The listing builds one solid part. Answer for the finished solid, in the listing's coordinates (mm). Face numbers are marked on the shaded views. A direction names the side the tool comes from. Round coordinates to 2 decimals unless told otherwise and drop trailing zeros. Write each loop counter-clockwise with the first axis right and the second up, starting at its lowest first coordinate (ties: lowest second). Pieces come first, ordered by that corner, then holes.
(1) For the marked faces 1 and 2, determine the directions among +Z, -Z, +X, -X, +Y, -Y from which every point of the face is accessible in a straight line to the end or side of a thin tool.
(2) Each of these flat-tipped pins is pushed along its axis until it touches: pin 1 Ø3 at (x, z) = (-27, -23.5) entering from -Y; pin 2 Ø1.5 at (x, y) = (-22.5, -10) entering from -Z; pin 3 Ø4 at (x, y) = (4.5, -9) entering from -Z; pin 4 Ø8 at (x, z) = (1.5, 0.5) entering from +Y. Where does it stop, or does it pass through?
(3) A cutting plane is placed at B-B, the plane x = 0. Give the vertices of the cut face in (y, z).
(4) A cutting plane is placed at D-D, the plane y = -12. Give the vertices of the cut face in (x, z).
(5) A cutting plane is placed at A-A, the plane z = 0. Give the vertices of the cut face in (x, y), and give its area (3 significant figures).
(6) Find the intervals of material crossed by probe 1 along X at (y, z) = (-2.5, 8); probe 2 along Y at (x, z) = (-21, 17); probe 3 along X at (y, z) = (1.25, -0.5), in increasing order.
(7) A cutting plane is placed at C-C, the plane y = -3. Give the vertices of the cut face in (x, z), and give its area (3 significant figures).
(8) The mould has two halves that part along X. Classify the marked faces 3, 4 and 5: +X half, -X half, draft (parallel to the pull), parting line (faces both ways), or undercut.
from build123d import *

# Parameters (mm, degrees)
CROQUIS1_R              = 35
SALIENTE_EXTRUIR1_DEPTH = 5
CROQUIS2_R              = 24.5
SALIENTE_EXTRUIR2_DEPTH = 15
CROQUIS3_R              = 6.85
SALIENTE_EXTRUIR3_DEPTH = 30
CROQUIS4_R              = 2
CORTAR_EXTRUIR1_DEPTH   = 10
MATRIZC1_COUNT          = 6
CORTAR_EXTRUIR2_START   = -30
CORTAR_EXTRUIR2_DEPTH   = 30
CUT_EXTRUDE1_START      = -40
CUT_EXTRUDE1_DEPTH      = 40
SKETCH2_R               = 5
CUT_EXTRUDE2_DEPTH      = 7
SKETCH3_R               = 3
CUT_EXTRUDE3_DEPTH      = 52.176166328


with BuildPart() as part:
    # Croquis1 → Saliente-Extruir1 (new body)
    with BuildSketch(Plane(origin=(0, 0, 0), x_dir=(1, 0, 0), z_dir=(0, 1, 0))):
        with Locations(Location((0, 0, 0), (0, 0, 270))):
            Circle(CROQUIS1_R)
    extrude(amount=SALIENTE_EXTRUIR1_DEPTH)

    # Croquis2 → Saliente-Extruir2 (add)
    with BuildSketch(Plane.XZ):
        with Locations(Location((0, 0, 0), (0, 0, 270))):
            Circle(CROQUIS2_R)
    extrude(amount=SALIENTE_EXTRUIR2_DEPTH)

    # Croquis3 → Saliente-Extruir3 (add)
    with BuildSketch(Plane.XZ.offset(15)):
        with Locations(Location((0, 0, 0), (0, 0, 270))):
            Circle(CROQUIS3_R)
    extrude(amount=SALIENTE_EXTRUIR3_DEPTH)

    # Croquis4 → Cortar-Extruir1 (cut)
    with BuildSketch(Plane(origin=(0, 5, 0), x_dir=(1, 0, 0), z_dir=(0, 1, 0))):
        with Locations(Location((0, 16, 0), (0, 0, 270))):
            Circle(CROQUIS4_R)
    cortar_extruir1 = extrude(amount=-CORTAR_EXTRUIR1_DEPTH, mode=Mode.SUBTRACT)

    # MatrizC1: Cortar-Extruir1 ×6 about axis
    matrizc1_axis = Axis((0, 0, 0), (0, 1, 0))
    for i in range(1, MATRIZC1_COUNT):
        add(cortar_extruir1.rotate(matrizc1_axis, i * 360 / MATRIZC1_COUNT), mode=Mode.SUBTRACT)

    # Croquis7 → Cortar-Extruir2 (cut)
    with BuildSketch(Plane.XZ.offset(45).offset(CORTAR_EXTRUIR2_START)):
        with BuildLine():
            Line((-6.37749951, 2.5), (-3.47749951, 2.5))
            Line((-3.47749951, 2.5), (-3.47749951, -2.5))
            Line((-3.47749951, -2.5), (-6.37749951, -2.5))
            ThreePointArc((-6.37749951, -2.5), (-6.85, 0), (-6.37749951, 2.5))
        make_face()
    extrude(amount=CORTAR_EXTRUIR2_DEPTH, mode=Mode.SUBTRACT)

    # Sketch1 → Cut-Extrude1 (cut)
    with BuildSketch(Plane.XZ.offset(45).offset(CUT_EXTRUDE1_START)):
        with BuildLine():
            Line((-6.37749951, -2.5), (-9.35, -2.5))
            Line((-9.35, -2.5), (-9.35, 2.5))
            Line((-9.35, 2.5), (-6.37749951, 2.5))
            ThreePointArc((-6.37749951, 2.5), (6.85, 0), (-6.37749951, -2.5))
        make_face()
    extrude(amount=CUT_EXTRUDE1_DEPTH, mode=Mode.SUBTRACT)

    # Sketch2 → Cut-Extrude2 (cut)
    with BuildSketch(Plane(origin=(0, 5, 0), x_dir=(1, 0, 0), z_dir=(0, 1, 0))):
        with Locations(Location((0, 0, 0), (0, 0, 270))):
            Circle(SKETCH2_R)
    extrude(amount=-CUT_EXTRUDE2_DEPTH, mode=Mode.SUBTRACT)

    # Sketch3 → Cut-Extrude3 (cut, through all)
    with BuildSketch(Plane(origin=(0, -2, 0), x_dir=(1, 0, 0), z_dir=(0, 1, 0))):
        with Locations(Location((0, 0, 0), (0, 0, 270))):
            Circle(SKETCH3_R)
    extrude(amount=-CUT_EXTRUDE3_DEPTH, mode=Mode.SUBTRACT)


solid = part.part
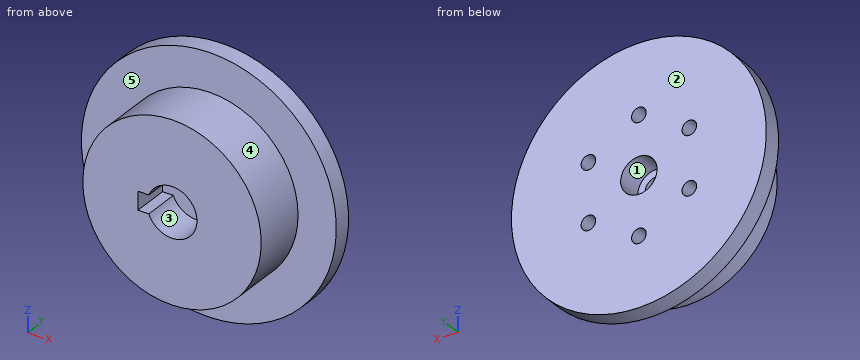
Solutions:
1. face 1: +Y
1. face 2: +Z, -Z, +X, -X, +Y
2. pin 1: stops at y = 0
2. pin 2: stops at z = -11.28
2. pin 3: stops at z = -24.37
2. pin 4: stops at y = 5
3. outline: (-15, -24.5) - (0, -24.5) - (0, -35) - (5, -35) - (5, -18) - (-5, -18) - (-5, -14) - (5, -14) - (5, -5) - (-2, -5) - (-2, -3) - (-5, -3) - (-5, -6.85) - (-15, -6.85) - close; (-15, 6.85) - (-5, 6.85) - (-5, 3) - (-2, 3) - (-2, 5) - (5, 5) - (5, 14) - (-5, 14) - (-5, 18) - (5, 18) - (5, 35) - (0, 35) - (0, 24.5) - (-15, 24.5) - close
4. outline: circle Ø49 at (0, 0); hole (-9.35, -2.5) - (-6.38, -2.5) arc R6.85 ccw (long way) to (-6.38, 2.5) - (-9.35, 2.5) - close
5. outline: (-35, 0) - (-24.5, 0) - (-24.5, -15) - (-9.35, -15) - (-9.35, -5) - (-3, -5) - (-3, -2) - (-5, -2) - (-5, 5) - (-35, 5) - close; (3, -5) - (6.85, -5) - (6.85, -15) - (24.5, -15) - (24.5, 0) - (35, 0) - (35, 5) - (5, 5) - (5, -2) - (3, -2) - close
5. area: 835 mm2
6. probe 1: x = -23.16 to -15.86, -11.86 to 11.86, 15.86 to 23.16
6. probe 2: y = 0 to 5
6. probe 3: x = -35 to -4.97, 4.97 to 35
7. outline: circle Ø49 at (0, 0); hole circle Ø4 at (-13.86, -8); hole circle Ø4 at (-13.86, 8); hole circle Ø6 at (0, 0); hole circle Ø4 at (0, -16); hole circle Ø4 at (0, 16); hole circle Ø4 at (13.86, -8); hole circle Ø4 at (13.86, 8)
7. area: 1,780 mm2
8. face 3: undercut
8. face 4: parting line
8. face 5: draft
